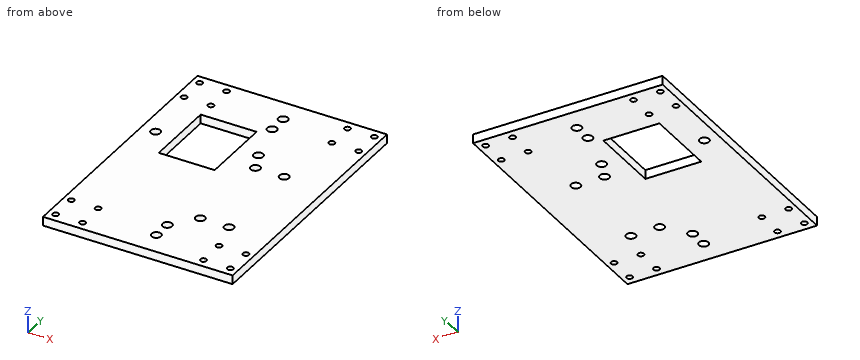
```python
from build123d import *

# Parameters (mm, degrees)
SKETCH1_W           = 127
SKETCH1_H           = 177.8
SKETCH1_R           = 2
SKETCH1_R_2         = 3.175
SKETCH1_W_2         = 37.465
SKETCH1_H_2         = 48.26
BOSS_EXTRUDE1_DEPTH = 5.9944


with BuildPart() as part:
    # Sketch1 → Boss-Extrude1 (new body)
    with BuildSketch(Plane.XY):
        with Locations((63.5, 88.9)):
            Rectangle(SKETCH1_W, SKETCH1_H)
        with Locations((5, 171.8)):
            Circle(SKETCH1_R, mode=Mode.SUBTRACT)
        with Locations((23, 171.8)):
            Circle(SKETCH1_R, mode=Mode.SUBTRACT)
        with Locations((5, 153.8)):
            Circle(SKETCH1_R, mode=Mode.SUBTRACT)
        with Locations((23, 153.8)):
            Circle(SKETCH1_R, mode=Mode.SUBTRACT)
        with Locations((104, 171.8)):
            Circle(SKETCH1_R, mode=Mode.SUBTRACT)
        with Locations((122, 171.8)):
            Circle(SKETCH1_R, mode=Mode.SUBTRACT)
        with Locations((104, 153.8)):
            Circle(SKETCH1_R, mode=Mode.SUBTRACT)
        with Locations((122, 153.8)):
            Circle(SKETCH1_R, mode=Mode.SUBTRACT)
        with Locations((23, 24)):
            Circle(SKETCH1_R, mode=Mode.SUBTRACT)
        with Locations((5, 24)):
            Circle(SKETCH1_R, mode=Mode.SUBTRACT)
        with Locations((5, 6)):
            Circle(SKETCH1_R, mode=Mode.SUBTRACT)
        with Locations((23, 6)):
            Circle(SKETCH1_R, mode=Mode.SUBTRACT)
        with Locations((122, 24)):
            Circle(SKETCH1_R, mode=Mode.SUBTRACT)
        with Locations((104, 24)):
            Circle(SKETCH1_R, mode=Mode.SUBTRACT)
        with Locations((104, 6)):
            Circle(SKETCH1_R, mode=Mode.SUBTRACT)
        with Locations((122, 6)):
            Circle(SKETCH1_R, mode=Mode.SUBTRACT)
        with Locations((98.7806, 44.45)):
            Circle(SKETCH1_R_2, mode=Mode.SUBTRACT)
        with Locations((79.5274, 44.45)):
            Circle(SKETCH1_R_2, mode=Mode.SUBTRACT)
        with Locations((79.5274, 107.95)):
            Circle(SKETCH1_R_2, mode=Mode.SUBTRACT)
        with Locations((98.7806, 107.95)):
            Circle(SKETCH1_R_2, mode=Mode.SUBTRACT)
        with Locations((9.6774, 113.03)):
            Circle(SKETCH1_R_2, mode=Mode.SUBTRACT)
        with Locations((74.0918, 120.65)):
            Circle(SKETCH1_R_2, mode=Mode.SUBTRACT)
        with Locations((66.675, 15.875)):
            Circle(SKETCH1_R_2, mode=Mode.SUBTRACT)
        with Locations((66.675, 161.925)):
            Circle(SKETCH1_R_2, mode=Mode.SUBTRACT)
        with Locations((66.675, 149.225)):
            Circle(SKETCH1_R_2, mode=Mode.SUBTRACT)
        with Locations((66.675, 28.575)):
            Circle(SKETCH1_R_2, mode=Mode.SUBTRACT)
        with Locations((41.5925, 118.11)):
            Rectangle(SKETCH1_W_2, SKETCH1_H_2, mode=Mode.SUBTRACT)
    extrude(amount=BOSS_EXTRUDE1_DEPTH)


solid = part.part
```
Input: part model. Units: mm. Frame: model coordinates. Coordinates: 2 decimals unless noted, no trailing zeros. Loops run counter-clockwise (first coordinate to the right, second up) from the corner with the lowest first, then second, coordinate; pieces in that order, holes last.
Q1. Section D-D, the plane z = 4.3. Give the number of separate pieces and of enclosed holes in the cut face, and give its area (3 significant figures).
Results are:
separate pieces: 1
enclosed holes: 27
area: 20,300 mm2
Q2. Section B-B, the plane x = 35.5. Return the cut outline in (y, z).
Results are:
outline: (0, 0) - (93.98, 0) - (93.98, 5.99) - (0, 5.99) - close; (142.24, 0) - (177.8, 0) - (177.8, 5.99) - (142.24, 5.99) - close
Q3. Section A-A, the plane y = 127. Return the cut outline in (x, z) (3 decimals).
Results are:
outline: (0, 0) - (22.86, 0) - (22.86, 5.994) - (0, 5.994) - close; (60.325, 0) - (127, 0) - (127, 5.994) - (60.325, 5.994) - close
Q4. Line query: line 1 along Y through (x, z) = (122, 4.6); line 2 along Y through (x, z) = (23, 3.1); line 3 along X through (y, z) = (171.8, 2.9). Output: solid intervals per line, ascending.
Results are:
line 1: y = 0 to 4, 8 to 22, 26 to 151.8, 155.8 to 169.8, 173.8 to 177.8
line 2: y = 0 to 4, 8 to 22, 26 to 93.98, 142.24 to 151.8, 155.8 to 169.8, 173.8 to 177.8
line 3: x = 0 to 3, 7 to 21, 25 to 102, 106 to 120, 124 to 127
Q5. Section C-C, the plane y = 44.45. Return the cut outline in (x, z), and give its area (3 significant figures).
Results are:
outline: (0, 0) - (76.35, 0) - (76.35, 5.99) - (0, 5.99) - close; (82.7, 0) - (95.61, 0) - (95.61, 5.99) - (82.7, 5.99) - close; (101.96, 0) - (127, 0) - (127, 5.99) - (101.96, 5.99) - close
area: 685 mm2
